```python
from build123d import *

# Parameters (mm, degrees)
BOSS_EXTRU_1_DEPTH             = 300
ENL_V_MAT_EXTRU_1_DEPTH        = 304.521004216
ENL_V_MAT_EXTRU_2_DEPTH        = 215.00934559
R_P_TITION_LIN_AIRE1_COUNT     = 8
R_P_TITION_LIN_AIRE1_PITCH     = 24
R_P_TITION_LIN_AIRE1_COL_COUNT = 8
R_P_TITION_LIN_AIRE1_COL_PITCH = 24


with BuildPart() as part:
    # Esquisse1 → Boss.-Extru.1 (new, symmetric)
    with BuildSketch(Plane.XY):
        Polygon((-10, 40), (-10, -5), (10, -5), (10, 0), (0, 0), (0, 40), align=None)
    extrude(amount=BOSS_EXTRU_1_DEPTH, both=True)

    # Esquisse2 → Enlèv. mat.-Extru.1 (cut, symmetric)
    with BuildSketch(Plane.XZ.offset(5)):
        Polygon((10, 190), (-10, 210), (-10, 300), (10, 300), align=None)
    enl_v_mat_extru_1 = extrude(amount=ENL_V_MAT_EXTRU_1_DEPTH, both=True, mode=Mode.SUBTRACT)

    # Symétrie1: Enlèv. mat.-Extru.1 across plane
    add(enl_v_mat_extru_1.mirror(Plane.XY), mode=Mode.SUBTRACT)

    # Esquisse3 → Enlèv. mat.-Extru.2 (cut, symmetric)
    with BuildSketch(Plane(origin=(0, 0, 0), x_dir=(0, 0, -1), z_dir=(1, 0, 0))):
        with BuildLine():
            Line((-4, 10), (-4, 30))
            ThreePointArc((-4, 30), (0, 34), (4, 30))
            Line((4, 30), (4, 10))
            ThreePointArc((4, 10), (0, 6), (-4, 10))
        make_face()
    enl_v_mat_extru_2 = extrude(amount=ENL_V_MAT_EXTRU_2_DEPTH, both=True, mode=Mode.SUBTRACT)

    # Répétition linéaire1: Enlèv. mat.-Extru.2 ×8
    with Locations(*[(0, 0, i * R_P_TITION_LIN_AIRE1_PITCH) for i in range(1, R_P_TITION_LIN_AIRE1_COUNT)]):
        add(enl_v_mat_extru_2, mode=Mode.SUBTRACT)

    # Répétition linéaire1 col: Enlèv. mat.-Extru.2 ×8
    with Locations(*[(0, 0, -i * R_P_TITION_LIN_AIRE1_COL_PITCH) for i in range(1, R_P_TITION_LIN_AIRE1_COL_COUNT)]):
        add(enl_v_mat_extru_2, mode=Mode.SUBTRACT)


solid = part.part
```
The listing builds one solid part. Answer for the finished solid, in the listing's coordinates (mm). Give positions to 0.01 mm unless a question says otherwise; leave off trailing zeros. Loops run counter-clockwise (first coordinate to the right, second up) from the corner with the lowest first, then second, coordinate; pieces in that order, holes last. Notation, with made-up numbers: M 35,35 L 41,35 A31 cw 41,72 Z; hole C 5,87 d6. An arc over 180 degrees is marked long. One line per item, written item: value.
1. For a pull along Y with two mould halves and no side action, classify faces 1 (the face through (0, -5, 3)), 2 (the face through (-5, 20, -116)), 3 (the face through (0, 33, 3)), 4 (the face through (-5, 6, -24)) as pulls with the +Y half, pulls with the -Y half, needs draft (parallel to the pull), parting line crosses it, or undercut.
Found:
face 1: pulls with the -Y half
face 2: undercut
face 3: needs draft
face 4: undercut
2. Section A-A on z = 72 is taken. Determine the outline of the cut face in (x, y).
Found:
outline: M -10,-5 L 10,-5 L 10,0 L 0,0 L 0,6 L -10,6 Z; M -10,34 L 0,34 L 0,40 L -10,40 Z
3. Section C-C on z = 158.5 is taken. Determine the outline of the cut face in (x, y), plus the area to 3 significant figures.
Found:
outline: M -10,-5 L 10,-5 L 10,0 L 0,0 L 0,40 L -10,40 Z
area: 500 mm^2
4. Each of these flat-tipped pins is pushed along its axis until it touches: P1, Ø8, axis at x = -5, y = 17, coming from the -Z side; P2, Ø10, axis at x = 4, y = 4, coming from the +Z side; P3, Ø8, axis at x = -4, y = 18, coming from the -Z side. Where does it stop, or does it pass through?
Found:
P1: z = -209
P2: z = 201
P3: z = -208
5. Section B-B on y = 24.5 is taken. State how many separate pieces and enclosed holes the cut face has, plus the area to 3 significant figures.
Found:
separate pieces: 16
enclosed holes: 0
area: 2,900 mm^2
6. Find the intervals of material crossed by probe 1 along Y at (x, z) = (7.75, 11); probe 2 along X at (y, z) = (2, -190); probe 3 along Z at (x, y) = (-8, 0), in increasing order.
Found:
probe 1: -5 to 0
probe 2: -10 to 0
probe 3: -208 to 208
7. Section D-D on x = 5.75 is taken. Determine the outline of the cut face in (y, z).
Found:
outline: M -5,-194.25 L 0,-194.25 L 0,194.25 L -5,194.25 Z
